```python
from build123d import *

# Parameters (mm, degrees)
SKETCH1_R           = 6.25
BOSS_EXTRUDE1_DEPTH = 14.5
SKETCH2_R           = 0.9
BOSS_EXTRUDE2_DEPTH = 11.1
SKETCH3_R           = 2.5
BOSS_EXTRUDE3_DEPTH = 5
SKETCH4_R           = 1.5
BOSS_EXTRUDE4_DEPTH = 5
BOSS_EXTRUDE5_START = 4
SKETCH5_R           = 0.9
BOSS_EXTRUDE5_DEPTH = 4
BOSS_EXTRUDE9_DEPTH = 4.5
CIRPATTERN1_COUNT   = 3


with BuildPart() as part:
    # Sketch1 → Boss-Extrude1 (new body)
    with BuildSketch(Plane(origin=(0, 0, 0), x_dir=(1, 0, 0), z_dir=(0, 1, 0))):
        with Locations(Location((0, 0, 0), (0, 0, 90))):
            Circle(SKETCH1_R)
    extrude(amount=BOSS_EXTRUDE1_DEPTH)

    # Sketch2 → Boss-Extrude2 (add)
    with BuildSketch(Plane(origin=(0, 0, 0), x_dir=(1, 0, 0), z_dir=(0, 1, 0))):
        with Locations(Location((0, 0, 0), (0, 0, 270))):
            Circle(SKETCH2_R)
    extrude(amount=-BOSS_EXTRUDE2_DEPTH)

    # Sketch3 → Boss-Extrude3 (add)
    with BuildSketch(Plane(origin=(0, 14.5, 0), x_dir=(1, 0, 0), z_dir=(0, 1, 0))):
        with Locations(Location((0, 0, 0), (0, 0, 270))):
            Circle(SKETCH3_R)
    extrude(amount=BOSS_EXTRUDE3_DEPTH)

    # Sketch4 → Boss-Extrude4 (add)
    with BuildSketch(Plane(origin=(0, 19.5, 0), x_dir=(1, 0, 0), z_dir=(0, 1, 0))):
        with Locations(Location((0, 0, 0), (0, 0, 270))):
            Circle(SKETCH4_R)
    extrude(amount=BOSS_EXTRUDE4_DEPTH)

    # Sketch5 → Boss-Extrude5 (add)
    with BuildSketch(Plane(origin=(0, 24.5, 0), x_dir=(1, 0, 0), z_dir=(0, 1, 0)).offset(BOSS_EXTRUDE5_START)):
        with Locations(Location((0, 0, 0), (0, 0, 270))):
            Circle(SKETCH5_R)
    extrude(amount=-BOSS_EXTRUDE5_DEPTH)

    # Sketch7 → Boss-Extrude9 (add)
    with BuildSketch(Plane(origin=(0, 14.5, 0), x_dir=(1, 0, 0), z_dir=(0, 1, 0))):
        with BuildLine():
            Line((-0.579481228, 2.431913137), (-1.495304536, 3.700729228))
            Line((-1.495304536, 3.700729228), (1.495304536, 3.700729228))
            Line((1.495304536, 3.700729228), (0.579481228, 2.431913137))
            ThreePointArc((0.579481228, 2.431913137), (0, 2.5), (-0.579481228, 2.431913137))
        make_face()
    boss_extrude9 = extrude(amount=BOSS_EXTRUDE9_DEPTH)

    # CirPattern1: Boss-Extrude9 ×3 about axis
    cirpattern1_axis = Axis((0, 0, 0), (0, 1, 0))
    for i in range(1, CIRPATTERN1_COUNT):
        add(boss_extrude9.rotate(cirpattern1_axis, i * 360 / CIRPATTERN1_COUNT))


solid = part.part
```
Could you check a few things on this model? Use its own coordinates, in mm. A direction names the side the tool comes from. Coordinates: 2 decimals unless noted, no trailing zeros. Write each loop counter-clockwise with the first axis right and the second up, starting at its lowest first coordinate (ties: lowest second). Pieces come first, ordered by that corner, then holes. Notation, with made-up numbers: (85.5, 44) -> (110.5, 44) arc R14 cw to (110.5, 57) -> close; hole circle Ø6 at (27.25, -16.75). An arc over 180 degrees is marked (long way). Write item = value, one per line. Start each with the question number.
(1) Will these pins go through, and if not, where does the flat tip stop? pin 1 (4 mm diameter, centred on x = 0, z = 3.5, fed in from -Y); pin 2 (1 mm diameter, centred on x = -0.5, z = -3, fed in from +Y); pin 3 (0.6 mm diameter, centred on x = -3.5, z = 2, fed in from +Y).
(2) We'd pull the mould along Z, two halves only. Please class faces 1 (the face through (2.8, 19, 1.6)), 2 (the face through (-0.345, 26.528, 0.831)), 3 (the face through (-1.031, 16.718, -3.057)): released by +Z, released by -Z, zero draft, split by the parting line, or undercut.
(3) I want a section at B-B (z = 0). Please give me the cut outline in (x, y).
(4) I want a section at D-D (z = -3.25). Please give me the cut outline in (x, y).
(5) Which directions (+Z, -Z, +X, -X, +Y, -Y) give clear straight access to the entire face, cutting with the end or side of a thin tool? Please do faces 4 (the face through (-0.345, -5.472, 0.831)), 5 (the face through (2.14, 16.72, 2.44)), 6 (the face through (-2, 19.5, 0)), 7 (the face through (-3.194, 16.718, 1.868)).
(6) I want a section at A-A (x = 0). Please give me the cut outline in (y, z).
(7) I need wall thicknesses on line 1 (Y direction, x = 5.25, z = 2.25); line 2 (Y direction, x = 2.25, z = -0.5); line 3 (X direction, y = 23, z = 0). Which ranges of each line are inside material? Lowest first, please. Write a range as [from, to].
(8) I want a section at C-C (y = -1.5). Please give me the cut outline in (x, z).
Result set:
q1.pin_1 = 0
q1.pin_2 = 19
q1.pin_3 = 14.5
q2.face_1 = zero draft
q2.face_2 = split by the parting line
q2.face_3 = undercut
q3.outline = (-6.25, 0) -> (-0.9, 0) -> (-0.9, -11.1) -> (0.9, -11.1) -> (0.9, 0) -> (6.25, 0) -> (6.25, 14.5) -> (2.5, 14.5) -> (2.5, 19.5) -> (1.5, 19.5) -> (1.5, 24.5) -> (0.9, 24.5) -> (0.9, 28.5) -> (-0.9, 28.5) -> (-0.9, 24.5) -> (-1.5, 24.5) -> (-1.5, 19.5) -> (-2.5, 19.5) -> (-2.5, 14.5) -> (-6.25, 14.5) -> close
q4.outline = (-5.34, 0) -> (5.34, 0) -> (5.34, 14.5) -> (1.17, 14.5) -> (1.17, 19) -> (-1.17, 19) -> (-1.17, 14.5) -> (-5.34, 14.5) -> close
q5.face_4 = -Y
q5.face_5 = +Z, +Y
q5.face_6 = +Y
q5.face_7 = +Z, -X, +Y
q6.outline = (-11.1, -0.9) -> (0, -0.9) -> (0, -6.25) -> (14.5, -6.25) -> (14.5, -3.7) -> (19, -3.7) -> (19, -2.5) -> (19.5, -2.5) -> (19.5, -1.5) -> (24.5, -1.5) -> (24.5, -0.9) -> (28.5, -0.9) -> (28.5, 0.9) -> (24.5, 0.9) -> (24.5, 1.5) -> (19.5, 1.5) -> (19.5, 2.5) -> (14.5, 2.5) -> (14.5, 6.25) -> (0, 6.25) -> (0, 0.9) -> (-11.1, 0.9) -> close
q7.line_1 = [0, 14.5]
q7.line_2 = [0, 19.5]
q7.line_3 = [-1.5, 1.5]
q8.outline = circle Ø1.8 at (0, 0)
